Here's the drawing with two shaded views (mm, measured from the low corner). I have some questions. A direction names the side the tool comes from. Coordinates: 2 decimals unless noted, no trailing zeros. Loops run counter-clockwise (first coordinate to the right, second up) from the corner with the lowest first, then second, coordinate; pieces in that order, holes last.
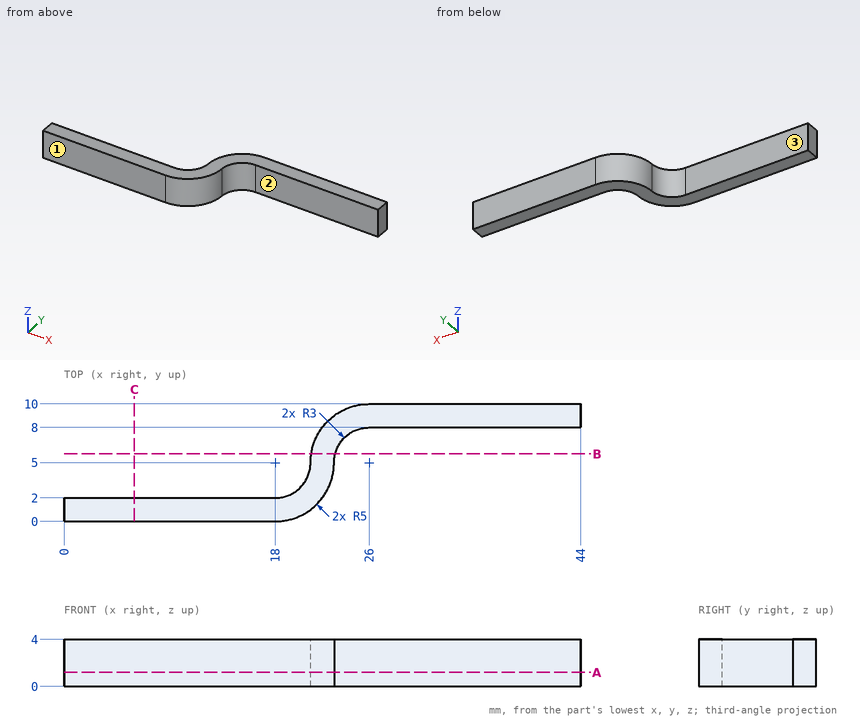
(1) I want a section at B-B on y = 5.75. Write out the boundary of the cut face in (x, z), then the cut area to 3 significant figures.
Check values:
outline: (21.06, 0) - (23.1, 0) - (23.1, 4) - (21.06, 4) - close
area: 8.15 mm2
(2) I want a section at A-A on z = 1.2. Write out the boundary of the cut face in (x, y), then the cut area to 3 significant figures.
Check values:
outline: (0, 0) - (18, 0) arc R5 ccw to (23, 5) arc R3 cw to (26, 8) - (44, 8) - (44, 10) - (26, 10) arc R5 ccw to (21, 5) arc R3 cw to (18, 2) - (0, 2) - close
area: 97.1 mm2
(3) I want a section at C-C on x = 6. Write out the boundary of the cut face in (y, z).
Check values:
outline: (0, 0) - (2, 0) - (2, 4) - (0, 4) - close
(4) If I drill on probe 1 along Y at (x, z) = (5, 2.2); probe 2 along Y at (x, z) = (38.5, 0.6); probe 3 along X at (y, z) = (1.5, 3.2), over which ranges is the centre line in solid material (lowest first)?
Check values:
probe 1: y = 0 to 2
probe 2: y = 8 to 10
probe 3: x = 0 to 21.57
(5) I'm going to push flat-ended pins straight in: pin 1 (5 mm diameter, centred on x = 22, y = 2, fed in from -Z); pin 2 (2 mm diameter, centred on x = 34, z = 2.5, fed in from -Y); pin 3 (1 mm diameter, centred on x = 12.5, z = 2.5, fed in from +Y). Where does each tip first touch, or does it pass through?
Check values:
pin 1: stops at z = 0
pin 2: stops at y = 8
pin 3: stops at y = 2
(6) Which directions (+Z, -Z, +X, -X, +Y, -Y) give clear straight access to the entire face, cutting with the end or side of a thin tool? Please do the marked faces 1, 2 and 3.
Check values:
face 1: +Z, -Z, +X, -X, -Y
face 2: +Z, -Z, +X, -Y
face 3: +Z, -Z, -X, +Y
